Model file for the job. Use its own axes, mm. Give positions to 0.01 mm unless a question says otherwise; leave off trailing zeros. Write each loop counter-clockwise with the first axis right and the second up, starting at its lowest first coordinate (ties: lowest second). Pieces come first, ordered by that corner, then holes.
```python
from build123d import *

# Parameters (mm, degrees)
BOSS_EXTRUDE1_DEPTH   = 60
F_2_5MM_DOWEL_HOLE1_D = 2.5


with BuildPart() as part:
    # Sketch1 → Boss-Extrude1 (new body)
    with BuildSketch(Plane(origin=(0, 0, 0), x_dir=(1, 0, 0), z_dir=(0, 1, 0))):
        with BuildLine():
            Line((0, 0), (0, 8.4))
            Line((0, 8.4), (-10.290849044, 8.4))
            Line((-10.290849044, 8.4), (-10.290849044, 7.4))
            ThreePointArc((-10.290849044, 7.4), (-6.718748073, 4.362554757), (-5, 0))
            Line((-5, 0), (0, 0))
        make_face()
    extrude(amount=BOSS_EXTRUDE1_DEPTH)

    # Ø2.5mm Dowel Hole1 (through all)
    with Locations(Plane(origin=(-2.5, 45, 0), x_dir=(1, 0, 0), z_dir=(0, 0, 1))):
        with Locations((0, 0), (0, -30)):
            Hole(F_2_5MM_DOWEL_HOLE1_D / 2)


solid = part.part
```
1. Probe probe 1 along Y at (x, z) = (-2.5, -2.75); probe 2 along Y at (x, z) = (-3.5, -0.5); probe 3 along Z at (x, y) = (-9, 55.5). List the from-to ranges inside material, lowest first.
Calculated:
probe 1: y = 0 to 13.75, 16.25 to 43.75, 46.25 to 60
probe 2: y = 0 to 14.25, 15.75 to 44.25, 45.75 to 60
probe 3: z = -8.4 to -6.63
2. Pull direction X, two halves, no side cores. Call faces 1 (the flat face through (0, 30, -4)), 2 (the cylindrical face through (-2.34, 46.24, -4.26)), 3 (the flat face through (-5, 30, -8.4)): +X half, -X half, draft (parallel to the pull), parting line (faces both ways), or undercut.
Calculated:
face 1: +X half
face 2: undercut
face 3: draft
3. Slice it at C-C, the plane z = -3. Write the cut outline in (x, y).
Calculated:
outline: (-5.9, 0) - (0, 0) - (0, 60) - (-5.9, 60) - close; hole circle Ø2.5 at (-2.5, 15); hole circle Ø2.5 at (-2.5, 45)
4. Slice it at D-D, the plane y = 37. Write the cut outline in (x, z).
Calculated:
outline: (-10.29, -8.4) - (0, -8.4) - (0, 0) - (-5, 0) arc R9.65 cw to (-10.29, -7.4) - close
5. Slice it at B-B, the plane y = 15. Write the cut outline in (x, z), and give its area (3 significant figures).
Calculated:
outline: (-10.29, -8.4) - (-3.75, -8.4) - (-3.75, 0) - (-5, 0) arc R9.65 cw to (-10.29, -7.4) - close; (-1.25, -8.4) - (0, -8.4) - (0, 0) - (-1.25, 0) - close
area: 38.9 mm2
6. Slice it at A-A, the plane x = -1.75. Write the cut outline in (y, z).
Calculated:
outline: (0, -8.4) - (14, -8.4) - (14, 0) - (0, 0) - close; (16, -8.4) - (44, -8.4) - (44, 0) - (16, 0) - close; (46, -8.4) - (60, -8.4) - (60, 0) - (46, 0) - close
7. Pin check, flat tips, straight feed: P1, Ø1, axis at y = 44.5, z = -4, coming from the -X side; P2, Ø1.5, axis at y = 53.5, z = -2, coming from the -X side. Stop position of each tip, or through.
Calculated:
P1: stops at x = -6.82
P2: stops at x = -5.79
